Geometry check sheet. Reference: the model listing, model coordinates, mm. A direction names the side the tool comes from. Round coordinates to 2 decimals unless told otherwise and drop trailing zeros. Loops run counter-clockwise (first coordinate to the right, second up) from the corner with the lowest first, then second, coordinate; pieces in that order, holes last. Notation, with made-up numbers: (30, 62) - (57, 62) arc R35 cw to (57, 97) - close; hole circle Ø3 at (5, -15). An arc over 180 degrees is marked (long way). Write item = value, one per line.
```python
from build123d import *

# Parameters (mm, degrees)
F0_W        = 53.6803901196
F0_H        = 98.2824712992
F1_DEPTH    = 8.89
F2_W        = 48.3321249485
F2_H        = 42.7858147305
F3_DEPTH    = 3.81
F4_T1_DEPTH = 48.3321249485
F4_T3_DEPTH = 55.0825368547


# Not quite as in the source:
# - a fillet or chamfer that OpenCascade refuses, or shapes differently, is made with other operations: its cross-section is extruded or revolved along the edge and cut away or added


with BuildPart() as f1:
    # F0 (on Top) → F1 (new body)
    with BuildSketch(Plane.XY):
        Rectangle(F0_W, F0_H)
    extrude(amount=-F1_DEPTH)

    # F2 (on Top) → F3 (cut)
    with BuildSketch(Plane.XY):
        with Locations((-0.504437834, 25.230371044)):
            Rectangle(F2_W, F2_H)
    extrude(amount=-F3_DEPTH, mode=Mode.SUBTRACT)

    # F4: fillet of radius 5.08 on 4 edges, made by hand

    # F4_s2 → F4_t1 (join)
    with BuildSketch(Plane.YZ.offset(-24.6705003083)):
        with BuildLine():
            ThreePointArc((46.6232784092, 0), (44.8154415329, -2.7460926284), (41.7045895596, -3.81))
            Line((41.7045895596, -3.81), (46.6232784092, -3.81))
            Line((46.6232784092, -3.81), (46.6232784092, 0))
        make_face()
        with BuildLine():
            ThreePointArc((3.8374636788, 0), (5.6453005551, -2.7460926284), (8.7561525285, -3.81))
            Line((8.7561525285, -3.81), (3.8374636788, -3.81))
            Line((3.8374636788, -3.81), (3.8374636788, 0))
        make_face()
    extrude(amount=F4_T1_DEPTH)

    # F4_s4 → F4_t3 (join)
    with BuildSketch(Plane.XZ.offset(-46.6232784092)):
        with BuildLine():
            ThreePointArc((-24.6705003083, 0), (-22.8626634319, -2.7460926284), (-19.7518114586, -3.81))
            Line((-19.7518114586, -3.81), (-24.6705003083, -3.81))
            Line((-24.6705003083, -3.81), (-24.6705003083, 0))
        make_face()
        with BuildLine():
            ThreePointArc((23.6616246402, 0), (21.8537877639, -2.7460926284), (18.7429357905, -3.81))
            Line((18.7429357905, -3.81), (23.6616246402, -3.81))
            Line((23.6616246402, -3.81), (23.6616246402, 0))
        make_face()
    extrude(amount=F4_T3_DEPTH)


solid = f1.part
```
(1) Set-up check for faces 1 (the cylindrical face through (-0.84, 5.61, -2.72)), 2 (the flat face through (0, 1, -8.89)): record each of +Z, -Z, +X, -X, +Y, -Y from which the full face is reachable in a straight line by a thin tool's end or side.
Answers follow:
face_1 = +Z
face_2 = -Z, +X, -X, +Y, -Y
(2) Section check B-B (y = 21). Enter the section's corners in (x, z).
Answers follow:
outline = (-26.84, -8.89) - (26.84, -8.89) - (26.84, 0) - (23.66, 0) arc R5.08 cw to (18.74, -3.81) - (-19.75, -3.81) arc R5.08 cw to (-24.67, 0) - (-26.84, 0) - close
(3) Section check C-C (z = -2.25). Enter the section's corners in (x, y), then the cut area to 3 significant figures.
Answers follow:
outline = (-26.84, -49.14) - (26.84, -49.14) - (26.84, 49.14) - (-26.84, 49.14) - close; hole (-23.41, 5.09) - (22.41, 5.09) - (22.41, 45.37) - (-23.41, 45.37) - close
area = 3,430 mm²
(4) Section check A-A (x = 1). Enter the section's corners in (y, z).
Answers follow:
outline = (-49.14, -8.89) - (49.14, -8.89) - (49.14, 0) - (46.62, 0) arc R5.08 cw to (41.7, -3.81) - (8.76, -3.81) arc R5.08 cw to (3.84, 0) - (-49.14, 0) - close
(5) Mould release check, pull along X, two halves, no side actions. Record for faces 3 (the cylindrical face through (-22.9, 25.53, -2.717)), 4 (the flat face through (26.84, -1, -4)), 5 (the cylindrical face through (-0.84, 44.85, -2.72)), 6 (the flat face through (0, 49.141, -4)): pulls with the +X half, pulls with the -X half, needs draft (parallel to the pull), parting line crosses it, or undercut.
Answers follow:
face_3 = undercut
face_4 = pulls with the +X half
face_5 = undercut
face_6 = needs draft
(6) Scan lines: L1, parallel to X at y = 18.5, z = -0.75; L2, parallel to Z at x = 2.5, y = 37; L3, parallel to Y at x = -3.5, z = -2.75. Record each from-to range of solid material in increasing order. Write a range as [from, to].
Answers follow:
L1 = [-26.84, -24.41], [23.4, 26.84]
L2 = [-8.89, -3.81]
L3 = [-49.14, 5.65], [44.81, 49.14]
